```python
from build123d import *

# Parameters (mm, degrees)
F1_R        = 5
F1_R_2      = 3.5
F2_DEPTH    = 30
F4_W        = 1.5
F4_H        = 2.639524132
F5_DEPTH    = 29.5
F6_COUNT    = 4
F8_R        = 3.5
F8_R_2      = 1.75
F9_DEPTH    = 1.5
F10_SIZE2   = 1.49999
F10_SIZE    = 9.99999
F10_2_SIZE2 = 1.49999
F10_2_SIZE  = 9.99999
F10_3_SIZE2 = 1.49999
F10_3_SIZE  = 9.99999
F10_4_SIZE2 = 1.49999
F10_4_SIZE  = 9.99999
F11_SIZE    = 0.5
F12_R       = 0.49999


# Not quite as in the source:
# - a fillet or chamfer is up to 0.001 mm smaller than in the source, because OpenCascade refuses the exact size


with BuildPart() as f2:
    # F1 (on offset) → F2 (new body)
    with BuildSketch(Plane.XY):
        with Locations((-25, 25)):
            Circle(F1_R)
        with Locations((-25, 25)):
            Circle(F1_R_2, mode=Mode.SUBTRACT)
    extrude(amount=-F2_DEPTH)

    # F4 (on offset) → F5 (join)
    with BuildSketch(Plane.XY):
        with Locations((-25, 30.180237934)):
            Rectangle(F4_W, F4_H)
    extrude(amount=-F5_DEPTH)

    # F6: F2 ×4 about axis
    f6_axis = Axis((-25, 25, 0), (0, 0, 1))


with BuildPart() as f2_1:
    add(f2.part)
    for i in range(1, F6_COUNT):
        add(f2.part.rotate(f6_axis, i * 360 / F6_COUNT))

    # F8 (on offset) → F9 (join)
    with BuildSketch(Plane.XY.offset(-30)):
        with Locations((-25, 25)):
            Circle(F8_R)
        with Locations((-25, 25)):
            Circle(F8_R_2, mode=Mode.SUBTRACT)
    extrude(amount=F9_DEPTH)

    # F10 (size 10 and 1.5 in the source; OpenCascade refuses exactly that, so slightly less here)
    f10_edges = [f2_1.edges().sort_by_distance(p)[0] for p in [
        (-25, 18.5, -29.5),
    ]]
    f10_side = f2_1.faces().sort_by_distance((-25, 18.5, -14.75))[0]
    chamfer(f10_edges, length=F10_SIZE, length2=F10_SIZE2, reference=f10_side)

    # F10#2 (size 10 and 1.5 in the source; OpenCascade refuses exactly that, so slightly less here)
    f10_2_edges = [f2_1.edges().sort_by_distance(p)[0] for p in [
        (-18.5, 25, -29.5),
    ]]
    f10_2_side = f2_1.faces().sort_by_distance((-18.5, 25, -14.75))[0]
    chamfer(f10_2_edges, length=F10_2_SIZE, length2=F10_2_SIZE2, reference=f10_2_side)

    # F10#3 (size 10 and 1.5 in the source; OpenCascade refuses exactly that, so slightly less here)
    f10_3_edges = [f2_1.edges().sort_by_distance(p)[0] for p in [
        (-25, 31.5, -29.5),
    ]]
    f10_3_side = f2_1.faces().sort_by_distance((-25, 31.5, -14.75))[0]
    chamfer(f10_3_edges, length=F10_3_SIZE, length2=F10_3_SIZE2, reference=f10_3_side)

    # F10#4 (size 10 and 1.5 in the source; OpenCascade refuses exactly that, so slightly less here)
    f10_4_edges = [f2_1.edges().sort_by_distance(p)[0] for p in [
        (-31.5, 25, -29.5),
    ]]
    f10_4_side = f2_1.faces().sort_by_distance((-31.5, 25, -14.75))[0]
    chamfer(f10_4_edges, length=F10_4_SIZE, length2=F10_4_SIZE2, reference=f10_4_side)

    # F11
    f11_edges = [f2_1.edges().sort_by_distance(p)[0] for p in [
        (-28.5, 25, 0),
        (-26.75, 25, -28.5),
    ]]
    chamfer(f11_edges, length=F11_SIZE)

    # F12 (radius 0.5 in the source; OpenCascade refuses exactly that, so slightly less here)
    f12_edges = [f2_1.edges().sort_by_distance(p)[0] for p in [
        (-30, 25, -30),
    ]]
    fillet(f12_edges, radius=F12_R)


solid = f2_1.part
```
Input: part model. Units: mm. Frame: model coordinates. A direction names the side the tool comes from. Round coordinates to 2 decimals unless told otherwise and drop trailing zeros. Loops run counter-clockwise (first coordinate to the right, second up) from the corner with the lowest first, then second, coordinate; pieces in that order, holes last. Notation, with made-up numbers: (2, 5.25) -> (27, 5.25) arc R24 cw to (27, 41.25) -> close; hole circle Ø2 at (-18, -34.75). An arc over 180 degrees is marked (long way). One line per item, written item: value.
(1) Section C-C (z = -22.75). Return the cut outline in (x, y).
Geometry check:
outline: (-31.01, 24.25) -> (-29.94, 24.25) arc R5 ccw to (-25.75, 20.06) -> (-25.75, 18.99) -> (-24.25, 18.99) -> (-24.25, 20.06) arc R5 ccw to (-20.06, 24.25) -> (-18.99, 24.25) -> (-18.99, 25.75) -> (-20.06, 25.75) arc R5 ccw to (-24.25, 29.94) -> (-24.25, 31.01) -> (-25.75, 31.01) -> (-25.75, 29.94) arc R5 ccw to (-29.94, 25.75) -> (-31.01, 25.75) -> close; hole circle Ø7 at (-25, 25)
(2) Mould query, pull axis Y, two halves, no side actions, for faces 6 (the face through (-21.66, 26.05, -14.3)), 7 (the face through (-25, 31.5, -10)), 8 (the face through (-20.381, 23.085, -14.544)). Classes: pulls with the +Y half, pulls with the -Y half, needs draft (parallel to the pull), parting line crosses it, or undercut.
Geometry check:
face 6: undercut
face 7: pulls with the +Y half
face 8: parting line crosses it
(3) Material intervals for line 1 (X direction, y = 25, z = -14.25); line 2 (Y direction, x = -25, z = -17); line 3 (Z direction, x = -22.75, y = 23.25), sorted ascending. Write a range as [from, to].
Geometry check:
line 1: [-31.5, -28.5], [-21.5, -18.5]
line 2: [18.5, 21.5], [28.5, 31.5]
line 3: [-30, -28.5]
(4) Pin query (flat end, axial travel): pin 1 (0.5 mm diameter, centred on y = 30.5, z = -8.5, fed in from -X); pin 2 (3 mm diameter, centred on y = 27.5, z = -12.5, fed in from +X); pin 3 (1.7 mm diameter, centred on x = -31, z = -18, fed in from +Y). Return the tip coordinate at first contact, or that it passes through.
Geometry check:
pin 1: x = -25.75
pin 2: x = -20.1
pin 3: y = 25.75
(5) Set-up query: faces 1 (the face through (-25.75, 19, -11)), 2 (the face through (-24.25, 19, -11)), 3 (the face through (-31, 25.75, -11)), 4 (the face through (-28, 22, 0)), 5 (the face through (-24.25, 31, -11)). Return all of +Z, -Z, +X, -X, +Y, -Y with unobstructed straight access to the full face (end or side cutting, diameter ignored); none if empty.
Geometry check:
face 1: +Z, -Z, -X, -Y
face 2: +Z, -Z, +X, -Y
face 3: +Z, -Z, -X, +Y
face 4: +Z, +X, -X, +Y, -Y
face 5: +Z, -Z, +X, +Y
(6) Section D-D (y = 30.5). Return the cut outline in (x, z), plus the area to 4 significant figures.
Geometry check:
outline: (-25.75, -26.17) -> (-24.25, -26.17) -> (-24.25, 0) -> (-25.75, 0) -> close
area: 39.25 mm2
